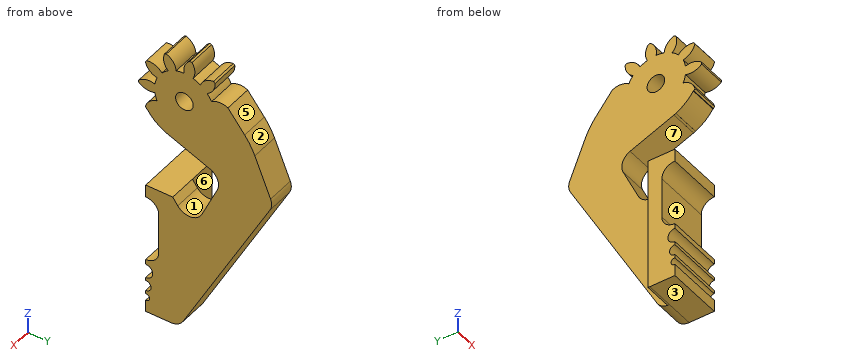
from build123d import *

# Parameters (mm, degrees)
BASPROSKE_W                 = 4
BASPROSKE_H                 = 6.5
TOOTHCUT_DEPTH              = 11.024968828
TEETHCUTS_COUNT             = 11
TEETHCUTS_ANGLE             = 327.272727273
BORSKE_R                    = 1.25
BORE_DEPTH                  = 62.5000635
Y_KSEKLIK_EKSTR_ZYON1_DEPTH = 4
Y_KSEKLIK_EKSTR_ZYON2_DEPTH = 4
RADYUS1_R                   = 10


with BuildPart() as part:
    # BasProSke → Base-Revolve (revolve)
    with BuildSketch(Plane(origin=(0, 0, 0), x_dir=(1, 0, 0), z_dir=(0, 1, 0)), mode=Mode.PRIVATE) as base_revolve_sk:
        with Locations((2, 3.25)):
            Rectangle(BASPROSKE_W, BASPROSKE_H)
    revolve(base_revolve_sk.sketch.rotate(Axis((-10, 0, 0), (1, 0, 0)), 180), axis=Axis((-10, 0, 0), (1, 0, 0)))

    # TooCutSke → ToothCut (cut, through all)
    with BuildSketch(Plane(origin=(0, 0, 0), x_dir=(0, 0, -1), z_dir=(1, 0, 0))):
        with BuildLine():
            ThreePointArc((0.576045815, 4.209771041), (0, 4.249), (-0.576045815, 4.209771041))
            ThreePointArc((-0.576045815, 4.209771041), (-0.841371334, 5.420048739), (-1.718652745, 6.295004202))
            ThreePointArc((-1.718652745, 6.295004202), (0, 6.5254), (1.718652745, 6.295004202))
            ThreePointArc((1.718652745, 6.295004202), (0.841371334, 5.420048739), (0.576045815, 4.209771041))
        make_face()
    toothcut = extrude(amount=TOOTHCUT_DEPTH, mode=Mode.SUBTRACT)

    # TeethCuts: ToothCut ×11 about axis
    teethcuts_axis = Axis((-10, 0, 0), (1, 0, 0))
    for i in range(1, TEETHCUTS_COUNT):
        add(toothcut.rotate(teethcuts_axis, i * TEETHCUTS_ANGLE / (TEETHCUTS_COUNT - 1)), mode=Mode.SUBTRACT)

    # BorSke → Bore (cut, symmetric)
    with BuildSketch(Plane(origin=(0, 0, 0), x_dir=(0, 0, -1), z_dir=(1, 0, 0))):
        with Locations(Location((0, 0, 0), (0, 0, 180))):
            Circle(BORSKE_R)
    extrude(amount=BORE_DEPTH, both=True, mode=Mode.SUBTRACT)

    # Çizim1 → Yükseklik-Ekstrüzyon1 (add)
    with BuildSketch(Plane(origin=(4, 0, 0), x_dir=(0, 0, -1), z_dir=(1, 0, 0))):
        with BuildLine():
            Line((2.760779628, -3.22987567), (1.236039076, 1.290267465))
            Line((1.236039076, 1.290267465), (-1.738987524, 3.876844515))
            ThreePointArc((-1.738987524, 3.876844515), (-2.188277705, 5.001068805), (-1.97474715, 6.192767854))
            Line((-1.97474715, 6.192767854), (2.120750073, 9.468090654))
            Line((2.120750073, 9.468090654), (8.9405865, 12.251804864))
            ThreePointArc((8.9405865, 12.251804864), (9.807212476, 12.397047884), (10.652448939, 12.156815828))
            Line((10.652448939, 12.156815828), (33.309678392, -0.173886099))
            ThreePointArc((33.309678392, -0.173886099), (34.072949781, -0.908840205), (34.353634969, -1.930582137))
            Line((34.353634969, -1.930582137), (34.353634969, -5.5))
            Line((34.353634969, -5.5), (32.660479675, -5.5))
            ThreePointArc((32.660479675, -5.5), (32.162954251, -4.950316473), (31.665428827, -5.5))
            Line((31.665428827, -5.5), (31.175724059, -5.5))
            ThreePointArc((31.175724059, -5.5), (30.425852071, -4.73614356), (29.675980082, -5.5))
            Line((29.675980082, -5.5), (29.219830425, -5.5))
            ThreePointArc((29.219830425, -5.5), (28.219830425, -4.5), (27.219830425, -5.5))
            Line((27.219830425, -5.5), (26.498039052, -5.5))
            ThreePointArc((26.498039052, -5.5), (25.955354116, -4.189842668), (24.645196784, -3.647157732))
            Line((24.645196784, -3.647157732), (18.851825021, -3.647157732))
            ThreePointArc((18.851825021, -3.647157732), (17.559352829, -4.192979175), (17.049350889, -5.5))
            Line((17.049350889, -5.5), (15.2413188, -5.5))
            Line((15.2413188, -5.5), (15.2413188, -1.657187873))
            Line((15.2413188, -1.657187873), (16.22148633, -0.944515231))
            ThreePointArc((16.22148633, -0.944515231), (17.0357361, 0.868792159), (15.883922648, 2.488795908))
            Line((15.883922648, 2.488795908), (11.157138105, 4.671882096))
            ThreePointArc((11.157138105, 4.671882096), (9.616505575, 4.728916331), (8.493027441, 3.673170916))
            Line((8.493027441, 3.673170916), (5.962652768, -2.587812197))
            ThreePointArc((5.962652768, -2.587812197), (4.998691965, -4.113179975), (3.652524478, -5.314762425))
            ThreePointArc((3.652524478, -5.314762425), (2.917345271, -4.39606094), (2.760779628, -3.22987567))
        make_face()
    extrude(amount=-Y_KSEKLIK_EKSTR_ZYON1_DEPTH)

    # Çizim2 → Yükseklik-Ekstrüzyon2 (add)
    with BuildSketch(Plane.ZY):
        with BuildLine():
            Line((-34.353634969, -1.930582137), (-34.353634969, -5.5))
            Line((-34.353634969, -5.5), (-32.660479675, -5.5))
            ThreePointArc((-32.660479675, -5.5), (-32.162954251, -4.950316473), (-31.665428827, -5.5))
            Line((-31.665428827, -5.5), (-31.175724059, -5.5))
            ThreePointArc((-31.175724059, -5.5), (-30.425852071, -4.73614356), (-29.675980082, -5.5))
            Line((-29.675980082, -5.5), (-29.219830425, -5.5))
            ThreePointArc((-29.219830425, -5.5), (-28.219830425, -4.5), (-27.219830425, -5.5))
            Line((-27.219830425, -5.5), (-26.498039052, -5.5))
            ThreePointArc((-26.498039052, -5.5), (-25.955354116, -4.189842668), (-24.645196784, -3.647157732))
            Line((-24.645196784, -3.647157732), (-18.851825021, -3.647157732))
            ThreePointArc((-18.851825021, -3.647157732), (-17.559352829, -4.192979175), (-17.049350889, -5.5))
            Line((-17.049350889, -5.5), (-15.2413188, -5.5))
            Line((-15.2413188, -5.5), (-15.2413188, -1.657187873))
            Line((-15.2413188, -1.657187873), (-34.334860745, -1.657187873))
            ThreePointArc((-34.334860745, -1.657187873), (-34.348935892, -1.793563074), (-34.353634969, -1.930582137))
        make_face()
    extrude(amount=Y_KSEKLIK_EKSTR_ZYON2_DEPTH)

    # Radyus1
    radyus1_edges = [part.edges().sort_by_distance(p)[0] for p in [
        (2, 9.468090654, -2.120750073),
    ]]
    fillet(radyus1_edges, radius=RADYUS1_R)


solid = part.part
Work out the finished part from the listing and answer in its coordinate system (mm). Face numbers are marked on the shaded views. A direction names the side the tool comes from. Round coordinates to 2 decimals unless told otherwise and drop trailing zeros. Write each loop counter-clockwise with the first axis right and the second up, starting at its lowest first coordinate (ties: lowest second). Pieces come first, ordered by that corner, then holes. Notation, with made-up numbers: (22.25, -11) - (29.25, -11) arc R11 cw to (29.25, 10) - close; hole circle Ø9 at (5, 49.25). An arc over 180 degrees is marked (long way). Answer in a Markdown table with one row per item. Add a question column.
1. A cutting plane is placed at A-A, the plane x = -3. Determine the outline of the cut face in (y, z).
2. The mould has two halves that part along Y. Classify the marked faces 1, 2, 3 and 4: +Y half, -Y half, draft (parallel to the pull), parting line (faces both ways), or undercut.
3. Find the intervals of material crossed by line 1 along Y through (x, z) = (-2.5, -20.5); line 2 along Z through (x, y) = (2.75, 3.5); line 3 along X through (y, z) = (2.75, -26.5), in increasing order. Write a range as from..to.
4. Given pin 1 (9.5 mm diameter, centred on y = 2, z = -18, fed in from -X); pin 2 (3 mm diameter, centred on x = 0, z = -21, fed in from -Y); pin 3 (0.5 mm diameter, centred on x = 1.5, z = -29.5, fed in from -Y); pin 4 (3 mm diameter, centred on x = 0, y = -4.5, fed in from +Z), each flat-ended and moving along its own axis, determine where each tip first touches the part or whether it passes through.
5. For the marked faces 5, 6 and 7, determine the directions among +Z, -Z, +X, -X, +Y, -Y from which every point of the face is accessible in a straight line to the end or side of a thin tool.
6. A cutting plane is placed at B-B, the plane y = 8. Determine the outline of the cut face in (x, z), and give its area (3 significant figures).
Worked out:
| question | item | result |
|---|---|---|
| 1 | outline | (-5.5, -34.35) - (-1.93, -34.35) arc R2 ccw to (-1.66, -34.33) - (-1.66, -15.24) - (-5.5, -15.24) - (-5.5, -17.05) arc R1.8 cw to (-3.65, -18.85) - (-3.65, -24.65) arc R1.85 cw to (-5.5, -26.5) - (-5.5, -27.22) arc R1 cw to (-5.5, -29.22) - (-5.5, -29.68) arc R0.75 cw (long way) to (-5.5, -31.18) - (-5.5, -31.67) arc R0.5 cw (long way) to (-5.5, -32.66) - close |
| 2 | face 1 | undercut |
| 2 | face 2 | +Y half |
| 2 | face 3 | draft |
| 2 | face 4 | -Y half |
| 3 | line 1 | -3.65..-1.66 |
| 3 | line 2 | -26.56..-13.69, -8.42..2.41, 2.94..4.85 |
| 3 | line 3 | 0..4 |
| 4 | pin 1 | x = -4 |
| 4 | pin 2 | y = -3.65 |
| 4 | pin 3 | y = -5.5 |
| 4 | pin 4 | z = 3.68 |
| 5 | face 5 | +Z, +X, -X, +Y |
| 5 | face 6 | +Z, -Z, -X, +Y |
| 5 | face 7 | +X, -X, -Y |
| 6 | outline | (0, -18.29) - (4, -18.29) - (4, -0.29) - (0, -0.29) - close |
| 6 | area | 72.0 mm^2 |
